Part model, mm, in its own coordinate system. Round coordinates to 2 decimals unless told otherwise and drop trailing zeros. Order: outer loops, then holes, each group sorted by start corner. A loop starts at its lowest first (then second) coordinate and runs counter-clockwise, first axis right, second up. Notation, with made-up numbers: (-36, 85) - (-14, 85) arc R23 cw to (-14, 118) - close; hole circle Ø10 at (-32.5, 84.25). An arc over 180 degrees is marked (long way). Answer as a JSON object with one key per item and string values.
```python
from build123d import *

# Parameters (mm, degrees)
F1_DEPTH = 1


with BuildPart() as f1:
    # F0 (on Front) → F1 (new body)
    with BuildSketch(Plane.XZ):
        with BuildLine():
            Line((0, 32.5), (0, 0))
            Line((0, 0), (37.5, 0))
            Line((37.5, 0), (37.5, 25.347329))
            ThreePointArc((37.5, 25.347329), (32.442298, 27.442298), (30.347329, 32.5))
            Line((30.347329, 32.5), (0, 32.5))
        make_face()
        with BuildLine():
            Line((37.5, 25.347329), (37.5, 0))
            Line((37.5, 0), (75, 0))
            Line((75, 0), (75, 32.5))
            Line((75, 32.5), (44.652671, 32.5))
            ThreePointArc((44.652671, 32.5), (42.557702, 27.442298), (37.5, 25.347329))
        make_face()
        with BuildLine():
            Line((0, 65), (0, 32.5))
            Line((0, 32.5), (30.347329, 32.5))
            ThreePointArc((30.347329, 32.5), (32.442298, 37.557702), (37.5, 39.652671))
            Line((37.5, 39.652671), (37.5, 65))
            Line((37.5, 65), (0, 65))
        make_face()
        with BuildLine():
            Line((44.652671, 32.5), (75, 32.5))
            Line((75, 32.5), (75, 65))
            Line((75, 65), (37.5, 65))
            Line((37.5, 65), (37.5, 39.652671))
            ThreePointArc((37.5, 39.652671), (42.557702, 37.557702), (44.652671, 32.5))
        make_face()
    extrude(amount=F1_DEPTH)


solid = f1.part
```
Item 1: Cut at B-B (z = 35). Write the cut outline in (x, y).
Taken from the geometry:
{"outline": "(0, -1) - (30.8, -1) - (30.8, 0) - (0, 0) - close; (44.2, -1) - (75, -1) - (75, 0) - (44.2, 0) - close"}
Item 2: Cut at A-A (y = -0.45). Write the cut outline in (x, z), plus the area to 3 significant figures.
Taken from the geometry:
{"outline": "(0, 0) - (75, 0) - (75, 65) - (0, 65) - close; hole (30.35, 32.5) arc R7.15 ccw to (37.5, 25.35) arc R7.15 ccw to (44.65, 32.5) arc R7.15 ccw to (37.5, 39.65) arc R7.15 ccw to start", "area": "4,710 mm2"}
Item 3: Probe L1, parallel to X at y = -0.1, z = 32; L2, parallel to X at y = -0.2, z = 28.5; L3, parallel to Z at x = 40.5, y = -0.1. List the from-to ranges inside material, lowest first. Write a range as from..to.
Taken from the geometry:
{"L1": "0..30.36, 44.64..75", "L2": "0..31.57, 43.43..75", "L3": "0..26.01, 38.99..65"}
